Build history of the part. All positions in model axes, mm. Face numbers are marked on the shaded views. Give positions to 0.01 mm unless a question says otherwise; leave off trailing zeros. Loops run counter-clockwise (first coordinate to the right, second up) from the corner with the lowest first, then second, coordinate; pieces in that order, holes last. Notation, with made-up numbers: (87, -37.75) -> (100, -37.75) arc R36 cw to (100, -3.75) -> close; hole circle Ø2 at (4.5, 50.25). An arc over 180 degrees is marked (long way). Answer in a Markdown table with one row per item. Add a question column.
from build123d import *

# Parameters (mm, degrees)
SKETCH1_W           = 12.7
SKETCH1_H           = 12.7
BOSS_EXTRUDE1_DEPTH = 80
SKETCH2_R           = 2
CUT_EXTRUDE1_DEPTH  = 82.991341006
CUT_EXTRUDE2_DEPTH  = 82.991341006
BOSS_EXTRUDE2_START = 17
SKETCH5_R           = 2
BOSS_EXTRUDE2_DEPTH = 17
SKETCH6_R           = 2
BOSS_EXTRUDE3_DEPTH = 17
SKETCH7_W           = 130
SKETCH7_H           = 130
BOSS_EXTRUDE4_DEPTH = 2
SKETCH8_W           = 130
SKETCH8_H           = 130
BOSS_EXTRUDE5_DEPTH = 2


with BuildPart() as part:
    # Sketch1 → Boss-Extrude1 (new body)
    with BuildSketch(Plane.XY):
        with Locations((6.35, 6.35)):
            Rectangle(SKETCH1_W, SKETCH1_H)
    extrude(amount=BOSS_EXTRUDE1_DEPTH)

    # Sketch2 → Cut-Extrude1 (cut, through all)
    with BuildSketch(Plane(origin=(0, 12.7, 0), x_dir=(1, 0, 0), z_dir=(0, 1, 0))):
        with Locations(Location((6.668720536, -5, 0), (0, 0, 270))):
            Circle(SKETCH2_R)
        with Locations(Location((6.668720536, -20, 0), (0, 0, 270))):
            Circle(SKETCH2_R)
        with Locations(Location((6.668720536, -60, 0), (0, 0, 270))):
            Circle(SKETCH2_R)
        with Locations(Location((6.668720536, -75, 0), (0, 0, 270))):
            Circle(SKETCH2_R)
    extrude(amount=-CUT_EXTRUDE1_DEPTH, mode=Mode.SUBTRACT)

    # Sketch4 → Cut-Extrude2 (cut, through all)
    with BuildSketch(Plane.ZY):
        with BuildLine():
            ThreePointArc((40, 2.727500863), (49.05, 6.35), (40, 9.972499137))
            ThreePointArc((40, 9.972499137), (30.95, 6.35), (40, 2.727500863))
        make_face()
    extrude(amount=-CUT_EXTRUDE2_DEPTH, mode=Mode.SUBTRACT)

    # Sketch5 → Boss-Extrude2 (add)
    with BuildSketch(Plane(origin=(0, 0, 0), x_dir=(1, 0, 0), z_dir=(0, 1, 0)).offset(BOSS_EXTRUDE2_START)):
        with Locations(Location((6.668720536, -20, 0), (0, 0, 270))):
            Circle(SKETCH5_R)
        with Locations(Location((6.668720536, -5, 0), (0, 0, 270))):
            Circle(SKETCH5_R)
    extrude(amount=-BOSS_EXTRUDE2_DEPTH)

    # Sketch6 → Boss-Extrude3 (add)
    with BuildSketch(Plane(origin=(0, 12.7, 0), x_dir=(1, 0, 0), z_dir=(0, 1, 0))):
        with Locations(Location((6.668720536, -75, 0), (0, 0, 270))):
            Circle(SKETCH6_R)
        with Locations(Location((6.668720536, -60, 0), (0, 0, 270))):
            Circle(SKETCH6_R)
    extrude(amount=-BOSS_EXTRUDE3_DEPTH)

    # Sketch7 → Boss-Extrude4 (add)
    with BuildSketch(Plane(origin=(0, 17, 0), x_dir=(1, 0, 0), z_dir=(0, 1, 0))):
        with Locations((6.35, -40)):
            Rectangle(SKETCH7_W, SKETCH7_H)
    extrude(amount=BOSS_EXTRUDE4_DEPTH)

    # Sketch8 → Boss-Extrude5 (add)
    with BuildSketch(Plane.XZ.offset(4.3)):
        with Locations((6.35, 40)):
            Rectangle(SKETCH8_W, SKETCH8_H)
    extrude(amount=BOSS_EXTRUDE5_DEPTH)


solid = part.part
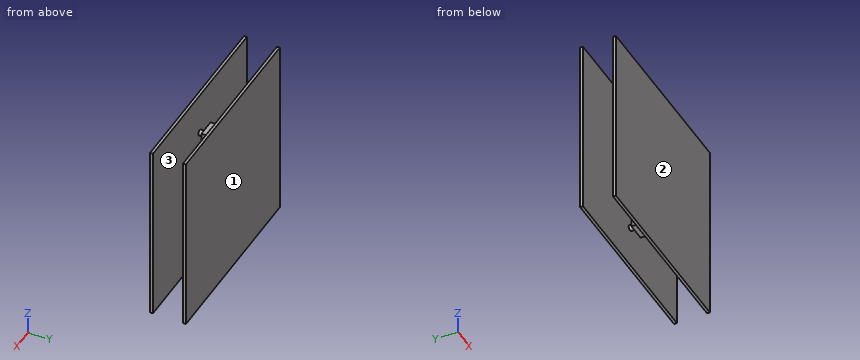
(1) Flat gauge pins, fed straight in: pin 1 Ø2 at (x, y) = (1, 6) entering from -Z; pin 2 Ø10 at (y, z) = (6, 23) entering from +X; pin 3 Ø4 at (y, z) = (9, 48) entering from -X; pin 4 Ø6 at (x, y) = (-39.5, 16) entering from +Z. Where does each tip first touch, or does it go through?
(2) Saw through at C-C, the plane z = 36.2. List the corners of the cut face in (x, y).
(3) Wall check: line 1 along Y through (x, z) = (9.75, 36.2); line 2 along Y through (x, z) = (-35, 41); line 3 along Y through (x, z) = (5, 43). Give the ranges that are in metal, low to high. Write a range as from..to.
(4) Saw through at A-A, the plane z = 81.5. List the corners of the cut face in (x, y), then the cut area to 3 significant figures.
(5) Saw through at B-B, the plane x = 57. List the corners of the cut face in (y, z), then the cut area to 3 significant figures.
(6) Saw through at D-D, the plane y = 14.5. List the corners of the cut face in (x, z).
(7) Two-plate mould, pull along Y, no slides. Class the marked faces 1, 2 and 3: released by +Y, released by -Y, zero draft, split by the parting line, or undercut.
Worked answers:
| question | item | result |
|---|---|---|
| 1 | pin 1 | z = 0 |
| 1 | pin 2 | x = 12.7 |
| 1 | pin 3 | x = 0 |
| 1 | pin 4 | z = 105 |
| 2 | outline | (-58.65, -6.3) -> (71.35, -6.3) -> (71.35, -4.3) -> (-58.65, -4.3) -> close; (-58.65, 17) -> (71.35, 17) -> (71.35, 19) -> (-58.65, 19) -> close; (0, 0) -> (12.7, 0) -> (12.7, 1.1) -> (0, 1.1) -> close; (0, 11.6) -> (12.7, 11.6) -> (12.7, 12.7) -> (0, 12.7) -> close |
| 3 | line 1 | -6.3..-4.3, 0..1.1, 11.6..12.7, 17..19 |
| 3 | line 2 | -6.3..-4.3, 17..19 |
| 3 | line 3 | -6.3..-4.3, 0..1.16, 11.54..12.7, 17..19 |
| 4 | outline | (-58.65, -6.3) -> (71.35, -6.3) -> (71.35, -4.3) -> (-58.65, -4.3) -> close; (-58.65, 17) -> (71.35, 17) -> (71.35, 19) -> (-58.65, 19) -> close |
| 4 | area | 520 mm^2 |
| 5 | outline | (-6.3, -25) -> (-4.3, -25) -> (-4.3, 105) -> (-6.3, 105) -> close; (17, -25) -> (19, -25) -> (19, 105) -> (17, 105) -> close |
| 5 | area | 520 mm^2 |
| 6 | outline | circle Ø4 at (6.67, 5); circle Ø4 at (6.67, 20) |
| 7 | face 1 | released by +Y |
| 7 | face 2 | released by -Y |
| 7 | face 3 | undercut |
